CAD build for the part. Positions are in the model's coordinates, mm. Face numbers are marked on the shaded views. A direction names the side the tool comes from. Coordinates: 2 decimals unless noted, no trailing zeros. Order: outer loops, then holes, each group sorted by start corner. A loop starts at its lowest first (then second) coordinate and runs counter-clockwise, first axis right, second up. Notation, with made-up numbers: (-35, 89) - (15, 89) arc R19 cw to (15, 116) - close; hole circle Ø1 at (87.25, 37). An arc over 180 degrees is marked (long way). Use one line per item in the form item = value.
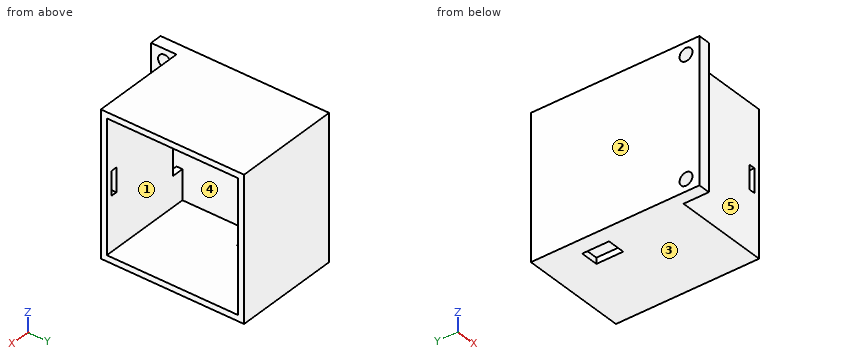
Autodesk Inventor part; units mm, degrees
ref_plane "YZ Plane" through (0, 0, 0) normal (1, 0, 0) x (0, 1, 0)
ref_plane "XZ Plane" through (0, 0, 0) normal (0, 1, 0) x (-1, 0, 0)
ref_plane "XY Plane" through (0, 0, 0) normal (0, 0, 1) x (1, 0, 0)
sketch "Sketch1" plane through (0, 0, 0) normal (1, 0, 0) x (0, 1, 0)
  line L0 (-38.1, 38.1) -> (38.1, 38.1)
  line L1 (38.1, 38.1) -> (38.1, -38.1)
  line L2 (38.1, -38.1) -> (-38.1, -38.1)
  line L3 (-38.1, -38.1) -> (-38.1, 38.1)
  line L4 (-38.1, 38.1) -> (0, 38.1)
  line L5 (-38.1, 34.925) -> (-38.1, 38.1)
  point P0 (0, 0)
  dimension "d0" = 76.2
  dimension "d1" = 76.2
  dimension "d2" = 38.1
  dimension "d3" = 38.1
extrude "Extrusion1" add sketch "Sketch1" along normal blind 6.35
sketch "Sketch2" plane through (6.35, 0, 0) normal (1, 0, 0) x (0, 0, -1)
  line L0 (-34.925, 34.925) -> (34.925, 34.925)
  line L1 (34.925, 34.925) -> (34.925, -34.925)
  line L2 (34.925, -34.925) -> (-34.925, -34.925)
  line L3 (-34.925, -34.925) -> (-34.925, 34.925)
  line L4 (38.1, 38.1) -> (-38.1, 38.1)
  line L5 (38.1, -38.1) -> (38.1, 38.1)
  line L6 (-38.1, 38.1) -> (-38.1, -38.1)
  line L7 (-38.1, -38.1) -> (38.1, -38.1)
  point P0 (0, 0)
  dimension "d6" = 3.175
  dimension "d7" = 3.175
  dimension "d8" = 3.175
  dimension "d9" = 3.175
extrude "Extrusion2" add sketch "Sketch2" along normal blind 50.8
sketch "Sketch4" plane through (0, -38.1, -38.1) normal (0, 0, -1) x (-1, 0, 0)
  line L0 (0, 0) -> (0, 76.2)
  line L1 (0, 76.2) -> (-57.15, 76.2)
  line L2 (-57.15, 0) -> (-57.15, 76.2)
  line L3 (0, 0) -> (-57.15, 0)
  line L4 (-6.35, 3.175) -> (-6.35, 73.025)
  line L5 (-8.4284, 41.2742) -> (-17.9534, 41.2742)
  line L6 (-17.9534, 41.2742) -> (-17.9534, 55.5617)
  line L7 (-17.9534, 55.5617) -> (-8.4284, 55.5617)
  line L8 (-8.4284, 55.5617) -> (-8.4284, 41.2742)
  point P0 (0, 38.1)
  dimension "d14" = 14.2875
  dimension "d15" = 9.525
extrude "Extrusion4" cut sketch "Sketch4" against normal blind 6.35 contours L5 L6 L7 L8
sketch "Sketch5" plane through (0, 0, 0) normal (-1, 0, 0) x (0, 0, 1)
  line L0 (-38.1, 38.1) -> (38.1, 38.1)
  line L1 (-38.1, -38.1) -> (-38.1, 38.1)
  line L2 (38.1, -38.1) -> (-38.1, -38.1)
  line L3 (38.1, 38.1) -> (38.1, -38.1)
  line L4 (38.1, -38.1) -> (-38.1, -38.1)
  line L5 (38.1, -38.1) -> (-38.1, -38.1)
  line L6 (-38.1, -38.1) -> (-38.1, -51.5938)
  line L7 (-38.1, -51.5938) -> (38.1, -51.5938)
  line L8 (38.1, -51.5938) -> (38.1, -38.1)
  circle A0 centre (31.75, -44.45) radius 3.429
  circle A1 centre (-31.75, -44.45) radius 3.429
  point P0 (0, 0)
  point P1 (0, -51.5938)
  dimension "d18" = 6.858
  dimension "d19" = 6.858
  dimension "d20" = 63.5
  dimension "d22" = 7.1437
  dimension "d23" = 7.1437
  dimension "d36" = 6.35
  dimension "d37" = 76.2
  dimension "d38" = 31.75
extrude "Extrusion5" add sketch "Sketch5" against normal blind 6.35 contours L2 L8 L7 L6
sketch "Sketch6" plane through (57.15, -38.1, -38.1) normal (0, -1, 0) x (1, 0, 0)
  line L0 (-50.8, 76.2) -> (-50.8, 0)
  line L1 (-50.8, 0) -> (0, 0)
  line L2 (0, 76.2) -> (0, 0)
  line L3 (-50.8, 76.2) -> (0, 76.2)
  line L4 (-57.15, 0) -> (-57.15, 76.2)
  line L5 (-57.15, 0) -> (-50.8, 0)
  line L6 (-50.8, 76.2) -> (-50.8, 0)
  line L7 (-57.15, 76.2) -> (-50.8, 76.2)
  line L8 (-50.8, 73.025) -> (-50.8, 3.175)
  line L9 (-50.8, 19.05) -> (-44.45, 19.05)
  line L10 (-44.45, 19.05) -> (-44.45, 57.15)
  line L11 (-44.45, 57.15) -> (-50.8, 57.15)
  line L12 (-50.8, 57.15) -> (-50.8, 19.05)
  line L13 (-6.35, 31.75) -> (-3.175, 31.75)
  line L14 (-3.175, 31.75) -> (-3.175, 44.45)
  line L15 (-3.175, 44.45) -> (-6.35, 44.45)
  line L16 (-6.35, 44.45) -> (-6.35, 31.75)
  point P0 (-57.15, 38.1)
  point P1 (-50.8, 38.1)
  point P2 (0, 38.1)
  dimension "d26" = 38.1
  dimension "d27" = 76.2
  dimension "d28" = 38.1
  dimension "d29" = 6.35
  dimension "d32" = 12.7
  dimension "d33" = 3.175
  dimension "d34" = 6.35
  dimension "d35" = 3.175
extrude "Extrusion6" cut sketch "Sketch6" against normal blind 14.2875 contours L11 L10 L9 L0 | L16 L15 L14 L13
equation "\"d7\" = d6"
equation "\"d8\" = d6"
equation "\"d9\" = d6"
equation "\"d19\" = d18"
equation "\"d22\" = d23"
properties part number "Part_1_box"
Item 1: Cut at D-D, the plane y = -44.45. Write the cut outline in (x, z), plus the area to 3 significant figures.
Derived:
outline = (0, -38.1) - (6.35, -38.1) - (6.35, -35.18) - (0, -35.18) - close; (0, -28.32) - (6.35, -28.32) - (6.35, 28.32) - (0, 28.32) - close; (0, 35.18) - (6.35, 35.18) - (6.35, 38.1) - (0, 38.1) - close
area = 397 mm²
Item 2: Drill centre lines: line 1 (Z direction, x = 23, y = 5) (3 decimals); line 2 (Y direction, x = 4.5, z = -31.75). Where is each one in solid material? Low to high. Write a range as [from, to].
Derived:
line_1 = [-38.1, -34.925], [34.925, 38.1]
line_2 = [-51.59, -47.88], [-41.02, 38.1]
Item 3: Cut at C-C, the plane y = 9. Write the cut outline in (x, z) (3 decimals), plus the area to 3 significant figures.
Derived:
outline = (0, -38.1) - (8.428, -38.1) - (8.428, -34.925) - (6.35, -34.925) - (6.35, 34.925) - (57.15, 34.925) - (57.15, 38.1) - (0, 38.1) - close; (17.953, -38.1) - (57.15, -38.1) - (57.15, -34.925) - (17.953, -34.925) - close
area = 776 mm²
Item 4: Drop flat-ended pins along their axis: pin 1 (4 mm diameter, centred on y = 19, z = 8, fed in from +X); pin 2 (1 mm diameter, centred on y = 9.5, z = -37, fed in from -X); pin 3 (2.5 mm diameter, centred on x = 11, z = -37, fed in from -Y). Give the stop position or say it passes through.
Derived:
pin_1 = 6.35
pin_2 = 0
pin_3 = -38.1
Item 5: Cut at B-B, the plane x = 45. Write the cut outline in (y, z) (3 decimals).
Derived:
outline = (-38.1, -38.1) - (38.1, -38.1) - (38.1, 38.1) - (-38.1, 38.1) - close; hole (-34.925, -34.925) - (34.925, -34.925) - (34.925, 34.925) - (-34.925, 34.925) - close
Item 6: Cut at A-A, the plane z = -31.75. Write the cut outline in (x, y) (3 decimals), plus the area to 3 significant figures.
Derived:
outline = (0, -51.594) - (6.35, -51.594) - (6.35, -47.879) - (0, -47.879) - close; (0, -41.021) - (6.35, -41.021) - (6.35, -38.1) - (57.15, -38.1) - (57.15, -34.925) - (6.35, -34.925) - (6.35, 34.925) - (57.15, 34.925) - (57.15, 38.1) - (0, 38.1) - close
area = 849 mm²
Item 7: Two-plate mould, pull along Y, no slides. Class the marked faces 3, 4 and 5: +Y half, -Y half, draft (parallel to the pull), parting line (faces both ways), or undercut.
Derived:
face_3 = draft
face_4 = undercut
face_5 = -Y half
Item 8: 3-axis set-ups, long thin cutter, end or side, ignore diameter. For the marked faces 1 and 2: which of +Z, -Z, +X, -X, +Y, -Y reach the whole face in a straight line?
Derived:
face_1 = +X
face_2 = +Z, -Z, -X, +Y, -Y
